Part model, mm, in its own coordinate system. Round coordinates to 2 decimals unless told otherwise and drop trailing zeros. Write each loop counter-clockwise with the first axis right and the second up, starting at its lowest first coordinate (ties: lowest second). Pieces come first, ordered by that corner, then holes.
1) Saw through at D-D on y = -24. Write the cut outline in (x, z), and give its area (3 significant figures).
2) Saw through at C-C on x = -7.5. Write the cut outline in (y, z), and give its area (3 significant figures).
3) Drill centre lines: L1, parallel to Y at x = -7, z = 5.9; L2, parallel to X at y = -24, z = 6.25; L3, parallel to X at y = -11.5, z = 6.35. Where is each one in solid material? Low to high.
4) Saw through at A-A on y = -11.5. Write the cut outline in (x, z).
5) Saw through at B-B on z = 5.9. Write the cut outline in (x, y).
6) Pull direction Y, two halves, no side cores. Call faces 1 (the cylindrical face through (-4.73, -12.65, 6.09)), 2 (the flat face through (10, -21, 6.6)), 3 (the flat face through (10, -39.399, 6)): +Y half, -Y half, draft (parallel to the pull), parting line (faces both ways), or undercut.
```python
from build123d import *

# Parameters (mm, degrees)
CYLINDER_R        = 3
CYLINDER_DEPTH    = 10
CYLINDER001_R     = 4
CYLINDER001_DEPTH = 10
SKETCH015_W       = 55.926
SKETCH015_H       = 35.3506
EXTRUDE034_DEPTH  = 1


with BuildPart() as cylinder:
    # Cylinder → Cylinder (new body)
    with BuildSketch(Plane(origin=(-7.5, -11.5, 4), x_dir=(1, 0, 0), z_dir=(0, 0, 1))):
        Circle(CYLINDER_R)
    extrude(amount=CYLINDER_DEPTH)


with BuildPart() as cylinder001:
    # Cylinder001 → Cylinder001 (new body)
    with BuildSketch(Plane(origin=(-10, -24, 4), x_dir=(1, 0, 0), z_dir=(0, 0, 1))):
        Circle(CYLINDER001_R)
    extrude(amount=CYLINDER001_DEPTH)


with BuildPart() as cut001:
    # Sketch015 (on Face6 of Extrude027) → Extrude034 (new body)
    with BuildSketch(Plane.XY.offset(5.6)):
        with Locations((10.249, -21.7237)):
            Rectangle(SKETCH015_W, SKETCH015_H)
    extrude(amount=EXTRUDE034_DEPTH)

    # Cut: cut Cylinder001
    add(cylinder001.part, mode=Mode.SUBTRACT)

    # Cut001: cut Cylinder
    add(cylinder.part, mode=Mode.SUBTRACT)


solid = cut001.part
```
Completed:
1. outline: (-17.71, 5.6) - (-14, 5.6) - (-14, 6.6) - (-17.71, 6.6) - close; (-6, 5.6) - (38.21, 5.6) - (38.21, 6.6) - (-6, 6.6) - close
1. area: 47.9 mm2
2. outline: (-39.4, 5.6) - (-27.12, 5.6) - (-27.12, 6.6) - (-39.4, 6.6) - close; (-20.88, 5.6) - (-14.5, 5.6) - (-14.5, 6.6) - (-20.88, 6.6) - close; (-8.5, 5.6) - (-4.05, 5.6) - (-4.05, 6.6) - (-8.5, 6.6) - close
2. area: 23.1 mm2
3. L1: y = -39.4 to -26.65, -21.35 to -14.46, -8.54 to -4.05
3. L2: x = -17.71 to -14, -6 to 38.21
3. L3: x = -17.71 to -10.5, -4.5 to 38.21
4. outline: (-17.71, 5.6) - (-10.5, 5.6) - (-10.5, 6.6) - (-17.71, 6.6) - close; (-4.5, 5.6) - (38.21, 5.6) - (38.21, 6.6) - (-4.5, 6.6) - close
5. outline: (-17.71, -39.4) - (38.21, -39.4) - (38.21, -4.05) - (-17.71, -4.05) - close; hole circle Ø8 at (-10, -24); hole circle Ø6 at (-7.5, -11.5)
6. face 1: undercut
6. face 2: draft
6. face 3: -Y half
